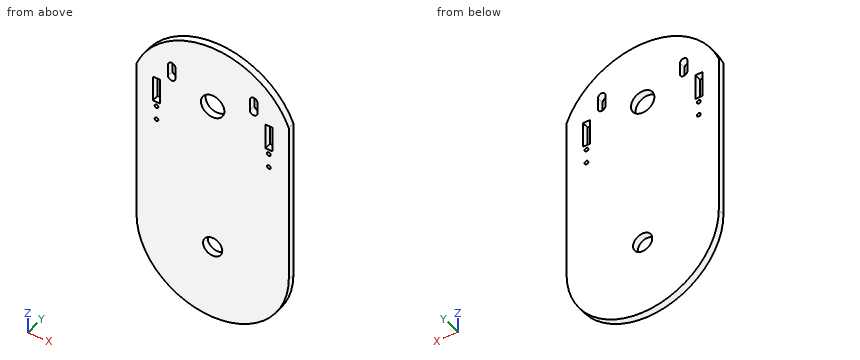
```python
from build123d import *

# Parameters (mm, degrees)
BOSS_EXTRUDE1_DEPTH = 3
SKETCH2_R           = 4.1
SKETCH2_R_2         = 5
SKETCH2_R_3         = 1.6
CUT_EXTRUDE1_DEPTH  = 4
SKETCH3_R           = 0.8
SKETCH3_W           = 3
SKETCH3_H           = 11
CUT_EXTRUDE2_DEPTH  = 4
CUT_EXTRUDE3_DEPTH  = 4


with BuildPart() as part:
    # Sketch1 → Boss-Extrude1 (new body)
    with BuildSketch(Plane(origin=(0, 0, 0), x_dir=(1, 0, 0), z_dir=(0, 1, 0))):
        with BuildLine():
            Line((-32.5, -35), (-32.5, 35))
            ThreePointArc((-32.5, 35), (0, 67.5), (32.5, 35))
            Line((32.5, 35), (32.5, -35))
            ThreePointArc((32.5, -35), (0, -57.009618943), (-32.5, -35))
        make_face()
    extrude(amount=BOSS_EXTRUDE1_DEPTH)

    # Sketch2 → Cut-Extrude1 (cut, through all)
    with BuildSketch(Plane(origin=(0, 3, 0), x_dir=(1, 0, 0), z_dir=(0, 1, 0))):
        with Locations((0, 35)):
            Circle(SKETCH2_R)
        with Locations((0, -30)):
            Circle(SKETCH2_R_2)
        with Locations((-17.5, -38)):
            Circle(SKETCH2_R_3)
        with Locations((17.5, -38)):
            Circle(SKETCH2_R_3)
    extrude(amount=-CUT_EXTRUDE1_DEPTH, mode=Mode.SUBTRACT)

    # Sketch3 → Cut-Extrude2 (cut, through all)
    with BuildSketch(Plane(origin=(0, 3, 0), x_dir=(1, 0, 0), z_dir=(0, 1, 0))):
        with Locations((-24, -13)):
            Circle(SKETCH3_R)
        with Locations((-24, -19)):
            Circle(SKETCH3_R)
        with Locations((24, -19)):
            Circle(SKETCH3_R)
        with Locations((24, -13)):
            Circle(SKETCH3_R)
        with Locations((24, -26.5)):
            Rectangle(SKETCH3_W, SKETCH3_H)
        with Locations((-24, -26.5)):
            Rectangle(SKETCH3_W, SKETCH3_H)
    extrude(amount=-CUT_EXTRUDE2_DEPTH, mode=Mode.SUBTRACT)

    # Sketch4 → Cut-Extrude3 (cut, through all)
    with BuildSketch(Plane(origin=(0, 3, 0), x_dir=(1, 0, 0), z_dir=(0, 1, 0))):
        with BuildLine():
            Line((-15.9, -35.5), (-15.9, -40.5))
            ThreePointArc((-15.9, -40.5), (-17.5, -42.1), (-19.1, -40.5))
            Line((-19.1, -40.5), (-19.1, -35.5))
            ThreePointArc((-19.1, -35.5), (-17.5, -33.9), (-15.9, -35.5))
        make_face()
        with BuildLine():
            Line((15.9, -35.5), (15.9, -40.5))
            ThreePointArc((15.9, -40.5), (17.5, -42.1), (19.1, -40.5))
            Line((19.1, -40.5), (19.1, -35.5))
            ThreePointArc((19.1, -35.5), (17.5, -33.9), (15.9, -35.5))
        make_face()
    extrude(amount=-CUT_EXTRUDE3_DEPTH, mode=Mode.SUBTRACT)


solid = part.part
```
The model under review builds one solid part; all positions refer to its coordinate system, in mm. Give positions to 0.01 mm unless a question says otherwise; leave off trailing zeros. Loops run counter-clockwise (first coordinate to the right, second up) from the corner with the lowest first, then second, coordinate; pieces in that order, holes last. Notation, with made-up numbers: (51, 23.25) - (82, 23.25) arc R22 cw to (82, 41.25) - close; hole circle Ø5 at (29.5, 64.5). An arc over 180 degrees is marked (long way). Answer as a JSON object with one key per item and string values.
Q1. Add section B-B on z = 30. State the section outline as (x, y) points, plus the area to 3 significant figures.
Worked out:
{"outline": "(-32.5, 0) - (-25.5, 0) - (-25.5, 3) - (-32.5, 3) - close; (-22.5, 0) - (-5, 0) - (-5, 3) - (-22.5, 3) - close; (5, 0) - (22.5, 0) - (22.5, 3) - (5, 3) - close; (25.5, 0) - (32.5, 0) - (32.5, 3) - (25.5, 3) - close", "area": "147 mm^2"}
Q2. Add section C-C on y = 1.2. Count the separate pieces of the cut face and the enclosed holes in it, plus the area to 3 significant figures.
Worked out:
{"separate pieces": "1", "enclosed holes": "10", "area": "6,990 mm^2"}
Q3. Add section A-A on x = 0. State the section outline as (y, z) points, plus the area to 3 significant figures.
Worked out:
{"outline": "(0, -67.5) - (3, -67.5) - (3, -39.1) - (0, -39.1) - close; (0, -30.9) - (3, -30.9) - (3, 25) - (0, 25) - close; (0, 35) - (3, 35) - (3, 57.01) - (0, 57.01) - close", "area": "319 mm^2"}
Q4. Insertion check: pin 1 (2.5 mm diameter, centred on x = -24, z = 13, fed in from +Y); pin 2 (0.9 mm diameter, centred on x = 23.5, y = 1, fed in from +Z); pin 3 (1 mm diameter, centred on x = -8.5, y = 2, fed in from +Z); pin 4 (1.4 mm diameter, centred on x = 24, z = 13, fed in from +Y). Each pin has a flat end and moves straight along its axis. Give the tip position at first contact, or say it passes through.
Worked out:
{"pin 1": "stops at y = 3", "pin 2": "stops at z = 48.35", "pin 3": "stops at z = 56.08", "pin 4": "passes through"}
Q5. Add section D-D on x = 17.5. State the section outline as (y, z) points.
Worked out:
{"outline": "(0, -62.39) - (3, -62.39) - (3, 33.9) - (0, 33.9) - close; (0, 42.1) - (3, 42.1) - (3, 52.32) - (0, 52.32) - close"}
Q6. To check wall thickness, follow line 1 along X through (y, z) = (1.05, 13); line 2 along X through (y, z) = (0.6, 30); line 3 along Z through (x, y) = (0, 2.1). State the ranges of each line that lie inside material, in increasing order.
Worked out:
{"line 1": "x = -32.5 to -24.8, -23.2 to 23.2, 24.8 to 32.5", "line 2": "x = -32.5 to -25.5, -22.5 to -5, 5 to 22.5, 25.5 to 32.5", "line 3": "z = -67.5 to -39.1, -30.9 to 25, 35 to 57.01"}
